Can you work these out from the model? Positions are in its coordinate system, mm. A direction names the side the tool comes from. Give positions to 0.01 mm unless a question says otherwise; leave off trailing zeros. Loops run counter-clockwise (first coordinate to the right, second up) from the corner with the lowest first, then second, coordinate; pieces in that order, holes last. Notation, with made-up numbers: M -6.75,3 L 24.25,3 A19 cw 24.25,9 Z; hole C -25,75.25 d3. An arc over 180 degrees is marked long. Put each result on its own line as item: value. Start each with the question number.
1) Imagine slicing it at A-A (x = 0). Write out the boundary of the cut face in (y, z), then the cut area to 3 significant figures.
2) Imagine slicing it at B-B (y = 22.5). Write out the boundary of the cut face in (x, z), then the cut area to 3 significant figures.
3) For faces 1 (the flat face through (-1.5, 3, 6)), 2 (the flat face through (4, 0, 4)), 3 (the flat face through (47, 9, 1)), 4 (the flat face through (3, 5, -6)), 5 (the flat face through (47.08, 6.48, 0.01)), which set-ups out of +Z, -Z, +X, -X, +Y, -Y let a thin tool reach every point of the face, with its end or its side?
4) For P1, Ø12, axis at y = 14.5, z = 41.5, coming from the +X side; P2, Ø2, axis at x = 36.5, y = 23.5, coming from the +Z side; P3, Ø2, axis at y = 19, z = 0.5, coming from the -X side; P4, Ø2, axis at x = 49.5, y = 6, coming from the +Z side, each with a flat end and sliding along its axis, tell me the tip position at first contact or that it passes through.
5) Imagine slicing it at D-D (x = 35). Write out the boundary of the cut face in (y, z), then the cut area to 3 significant figures.
6) Imagine slicing it at C-C (z = 16). Write out the boundary of the cut face in (x, y).
7) Please list where these lines run through material, in increasing order: line 1 along Y through (x, z) = (62, 25); line 2 along Z through (x, y) = (67.5, 19.75); line 3 along Y through (x, z) = (7.5, -11.5). Write a range as from..to.
8) If we mould it in two halves opening along Z, with no side actions, what happens to faces 6 (the flat face through (6, 0.006, 21)), 7 (the flat face through (-6, 3, 1.5)), 8 (the flat face through (47, 9, -1))? For each: +Z half, -Z half, draft (parallel to the pull), parting line (faces both ways), or undercut.
from build123d import *

# Parameters (mm, degrees)
SKETCH1_R           = 20
BOSS_EXTRUDE1_DEPTH = 5
BOSS_EXTRUDE2_DEPTH = 1
CIRPATTERN1_COUNT   = 2
CIRPATTERN1_ANGLE   = 75
CIRPATTERN3_COUNT   = 2
CIRPATTERN3_ANGLE   = 75
CUT_EXTRUDE1_REACH  = 7
BOSS_EXTRUDE3_DEPTH = 3.175


with BuildPart() as part:
    # Sketch1 → Boss-Extrude1 (new body)
    with BuildSketch(Plane(origin=(0, 0, 0), x_dir=(1, 0, 0), z_dir=(0, 1, 0))):
        Circle(SKETCH1_R)
    extrude(amount=BOSS_EXTRUDE1_DEPTH)

    # Sketch2 → Boss-Extrude2 (add, symmetric)
    with BuildSketch(Plane.XY):
        Polygon((19.75, 5), (26.1, 5), (66.58195138, 15.84710618), (66.58195138, 24.207798228), (70.58195138, 24.207798228), (70.58195138, 12.777798228), (22.917269596, 0.006085237), (19.75, 0.006085237), align=None)
    boss_extrude2 = extrude(amount=BOSS_EXTRUDE2_DEPTH, both=True)

    # CirPattern1: Boss-Extrude2 ×2 about axis
    cirpattern1_axis = Axis((0, 5, 0), (0, 1, 0))
    for i in range(1, CIRPATTERN1_COUNT):
        add(boss_extrude2.rotate(cirpattern1_axis, i * CIRPATTERN1_ANGLE / (CIRPATTERN1_COUNT - 1)))

    # CirPattern3: Boss-Extrude2 ×2 about axis
    cirpattern3_axis = Axis((0, 0, 0), (0, -1, 0))
    for i in range(1, CIRPATTERN3_COUNT):
        add(boss_extrude2.rotate(cirpattern3_axis, i * CIRPATTERN3_ANGLE / (CIRPATTERN3_COUNT - 1)))

    # Sketch5 → Cut-Extrude1 (cut, up to next)
    with BuildSketch(Plane(origin=(0, 5, 0), x_dir=(1, 0, 0), z_dir=(0, 1, 0)), mode=Mode.PRIVATE) as cut_extrude1_sk1:
        Polygon((-11, -1.5), (-1.5, -1.5), (-1.5, -11), (1.5, -11), (1.5, -1.5), (11, -1.5), (11, 1.5), (1.5, 1.5), (1.5, 11), (-1.5, 11), (-1.5, 1.5), (-11, 1.5), align=None)
    cut_extrude1_tool1 = extrude(cut_extrude1_sk1.sketch, amount=-CUT_EXTRUDE1_REACH, mode=Mode.PRIVATE) & part.part
    add(cut_extrude1_tool1.solids().sort_by_distance((0, 5, 0))[0], mode=Mode.SUBTRACT)

    # Sketch7 → Boss-Extrude3 (add)
    with BuildSketch(Plane(origin=(0, 24.207798228, 0), x_dir=(1, 0, 0), z_dir=(0, 1, 0))):
        with BuildLine():
            Line((17.302027431, 68.435748753), (16.266751251, 64.572045448))
            ThreePointArc((16.266751251, 64.572045448), (66.589460499, 0), (16.266751251, -64.572045448))
            Line((16.266751251, -64.572045448), (17.302027431, -68.435748753))
            ThreePointArc((17.302027431, -68.435748753), (70.589034988, 0), (17.302027431, 68.435748753))
        make_face()
    extrude(amount=BOSS_EXTRUDE3_DEPTH)


solid = part.part
Recorded:
1. outline: M 0,-20 L 5,-20 L 5,-11 L 0,-11 Z; M 0,11 L 5,11 L 5,20 L 0,20 Z
1. area: 90.0 mm²
2. outline: M 16.27,-64.57 L 17.3,-68.44 L 19.23,-67.92 L 18.2,-64.05 Z; M 16.27,64.57 L 18.2,64.05 L 19.23,67.92 L 17.3,68.44 Z; M 66.58,-1 L 70.58,-1 L 70.58,1 L 66.58,1 Z
2. area: 24.0 mm²
3. face 1: +Y, -Y
3. face 2: +Z, -Z, +X, -X, -Y
3. face 3: +Z, +X, -Y
3. face 4: -X, +Y
3. face 5: +Z, -Z, +X, -Y
4. P1: x = 13.45
4. P2: z = 60.84
4. P3: x = 66.58
4. P4: through
5. outline: M 3.24,-1 L 7.38,-1 L 7.38,1 L 3.24,1 Z; M 24.21,-61.3 L 27.38,-61.3 L 27.38,-56.65 L 24.21,-56.65 Z; M 24.21,56.65 L 27.38,56.65 L 27.38,61.3 L 24.21,61.3 Z
5. area: 37.8 mm²
6. outline: M -12,0 L 12,0 L 12,5 L -12,5 Z; M 64.64,24.21 L 68.75,24.21 L 68.75,27.38 L 64.64,27.38 Z
7. line 1: 24.21..27.38
7. line 2: -1..1
7. line 3: 0..5
8. face 6: draft
8. face 7: undercut
8. face 8: -Z half
